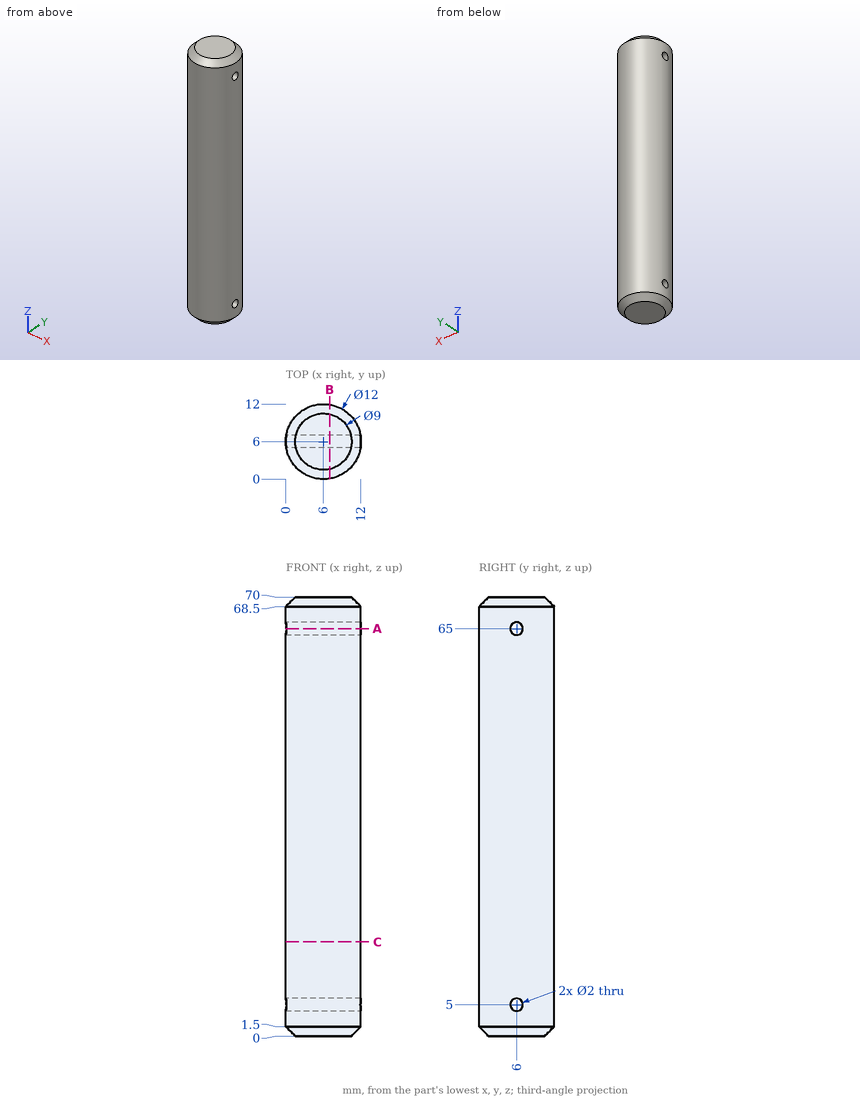
For this review, use the dimensioned drawing (mm, ordinates from the lowest corner) and the shaded views. Coordinates: 2 decimals unless noted, no trailing zeros. Loops run counter-clockwise (first coordinate to the right, second up) from the corner with the lowest first, then second, coordinate; pieces in that order, holes last.
1. For line 1 (Z direction, x = 3.5, y = 6.25); line 2 (Y direction, x = 3.25, z = 26); line 3 (Y direction, x = 5.5, z = 65), list the stretches that pass through material, from the lowest coordinate up.
2. Add section A-A, the plane z = 65. Give the boundary of the cut face in (x, y), then the cut area to 3 significant figures.
3. Add section C-C, the plane z = 15. Give the boundary of the cut face in (x, y), then the cut area to 3 significant figures.
4. Add section B-B, the plane x = 7. Count the separate pieces of the cut face and the enclosed holes in it, then the cut area to 3 significant figures.
5. Insertion check: P1, Ø2.5, axis at y = 6, z = 5, coming from the -X side; P2, Ø1, axis at x = 3.5, z = 19, coming from the +Y side; P3, Ø1.5, axis at y = 3.5, z = 15.5, coming from the +X side; P4, Ø3, axis at y = 3.5, z = 25.5, coming from the -X side. Each pin has a flat end and moves straight along its axis. Give the tip position at first contact, or say it passes through.
Result:
1. line 1: z = 0 to 4.03, 5.97 to 64.03, 65.97 to 70
1. line 2: y = 0.67 to 11.33
1. line 3: y = 0.02 to 5, 7 to 11.98
2. outline: (0.08, 5) arc R6 ccw to (11.92, 5) - close; (0.08, 7) - (11.92, 7) arc R6 ccw to start
2. area: 89.2 mm2
3. outline: circle Ø12 at (6, 6)
3. area: 113 mm2
4. separate pieces: 1
4. enclosed holes: 2
4. area: 817 mm2
5. P1: stops at x = 0
5. P2: stops at y = 11.66
5. P3: stops at x = 11.74
5. P4: stops at x = 0.08
